Input: part model. Units: mm. Frame: model coordinates. Face numbers are marked on the shaded views. Round coordinates to 2 decimals unless told otherwise and drop trailing zeros. Order: outer loops, then holes, each group sorted by start corner. A loop starts at its lowest first (then second) coordinate and runs counter-clockwise, first axis right, second up. Notation, with made-up numbers: (17.25, -31.75) -> (44.25, -31.75) arc R16 cw to (44.25, -20.75) -> close; hole circle Ø11 at (-6.75, 20). An arc over 180 degrees is marked (long way). Answer as CSV lines item,"result". Start each with the question number.
1) Section query C-C, the plane x = 0. Output: boundary loops of the cut face in (y, z).
2) Section query A-A, the plane y = 2.75. Output: boundary loops of the cut face in (x, z).
3) Section query D-D, the plane z = 12. Output: boundary loops of the cut face in (x, y), and give its area (3 significant figures).
4) Line query: L1, parallel to Y at x = 0, z = -11.5; L2, parallel to Z at x = 0, y = -1; L3, parallel to X at y = 4.75, z = 15. Output: solid intervals per line, ascending.
5) Mould query, pull axis X, two halves, no side actions, for the marked faces 1, 2, 3 and 4. Classes: +X half, -X half, draft (parallel to the pull), parting line (faces both ways), or undercut.
6) Section query B-B, the plane z = -5.5. Output: boundary loops of the cut face in (x, y), and give its area (3 significant figures).
7) First-contact query: P1, Ø2, axis at x = 0.5, y = 1, coming from the -Z side; P2, Ø6.5, axis at x = 0, z = 15, coming from the -Y side. Flat tips, straight axial feed; report the tip coordinate or a pass-through.
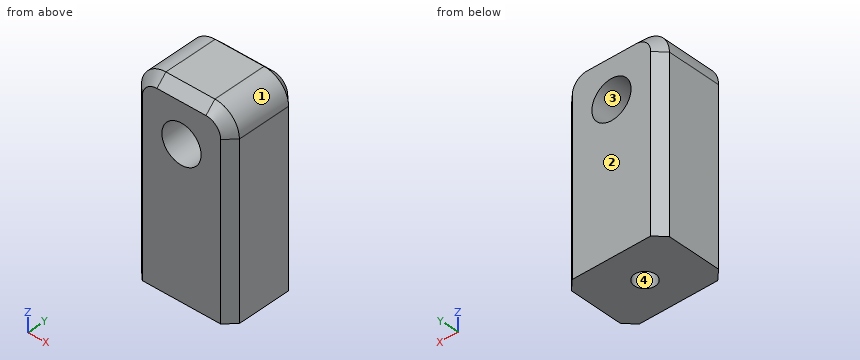
Autodesk Inventor part; units mm, degrees
ref_plane "YZ Plane" through (0, 0, 0) normal (1, 0, 0) x (0, 1, 0)
ref_plane "XZ Plane" through (0, 0, 0) normal (0, 1, 0) x (-1, 0, 0)
ref_plane "XY Plane" through (0, 0, 0) normal (0, 0, 1) x (1, 0, 0)
sketch "Sketch1" plane through (0, 0, 0) normal (0, 0, 1) x (1, 0, 0)
  line L0 (10, -7.5) -> (-10, -7.5)
  line L1 (-10, -7.5) -> (-10, 7.5)
  line L2 (-10, 7.5) -> (10, 7.5)
  line L3 (10, 7.5) -> (10, -7.5)
  line L4 (10, -7.5) -> (-10, 7.5) construction
  line L5 (-10, -7.5) -> (10, 7.5) construction
  line L6 (-10, 7.5) -> (10, 7.5)
  line L7 (10, 7.5) -> (10, 13.5)
  line L8 (10, 13.5) -> (-10, 13.5)
  line L9 (-10, 13.5) -> (-10, 7.5)
  line L10 (-10, -7.5) -> (10, -7.5)
  line L11 (10, -7.5) -> (10, -13.5)
  line L12 (10, -13.5) -> (-10, -13.5)
  line L13 (-10, -13.5) -> (-10, -7.5)
  point P0 (0, 0)
  dimension "d0" = 15
  dimension "d1" = 20
  dimension "d2" = 6
extrude "Extrusion1" add sketch "Sketch1" against normal blind 15
extrude "Extrusion2" add sketch "Sketch1" along normal blind 25 contours L11 L12 L13 L0 | L2 L9 L8 L7
sketch "Sketch2" plane through (-10, 13.5, -15) normal (0, 1, 0) x (1, 0, 0)
  line L0 (20, -15) -> (0, -15)
  line L1 (20, -40) -> (0, -40) construction
  line L2 (10, -40) -> (10, -30) construction
  circle A0 centre (10, -30) radius 4
  point P0 (10, -15)
  dimension "d7" = 8
  dimension "d8" = 10
extrude "Extrusion3" cut sketch "Sketch2" against normal through all
fillet "Fillet1" radius 5 4 edges at (-10, 10.5, 25) (10, 10.5, 25) (-10, -10.5, 25) (10, -10.5, 25)
sketch "Sketch3" plane through (0, 0, -15) normal (0, 0, -1) x (-1, 0, 0)
  circle A0 centre (0, 0) radius 2.15
  dimension "d12" = 4.3
extrude "Extrusion4" cut sketch "Sketch3" against normal through all
chamfer "Chamfer1" distance 2 angle 45 6 edges at (8.5355, 13.5, 23.5355) (0, 13.5, 25) (-8.5355, 13.5, 23.5355) (8.5355, -13.5, 23.5355) (0, -13.5, 25) (-8.5355, -13.5, 23.5355)
chamfer "Chamfer2" distance 4 angle 45 1 edges at (-10, 0, 0)
sketch "Sketch4" plane through (-5, 7.5, 25) normal (0, -1, 0) x (1, 0, 0)
  circle A0 centre (5, -10) radius 4
  arc A1 (15, -5) -> (10, 0) centre (10, -5) ccw
  line L0 (0, 0) -> (10, 0)
  arc A2 (0, 0) -> (-5, -5) centre (0, -5) ccw
  line L1 (-5, -29) -> (-5, -5)
  line L2 (-1, -25) -> (-5, -29)
  line L3 (15, -25) -> (-1, -25)
  line L4 (15, -25) -> (15, -5)
  point P0 (5, -25)
extrude "Extrusion5" add sketch "Sketch4" along normal up to next
sketch "Sketch5" plane through (0, 0, -15) normal (0, 0, -1) x (-1, 0, 0)
  line L0 (10, -11.5) -> (8, -13.5)
  line L1 (10, -11.5) -> (10, 11.5)
  line L2 (8, 13.5) -> (10, 11.5)
  line L3 (8, 13.5) -> (-8, 13.5)
  line L4 (-10, 11.5) -> (-8, 13.5)
  line L5 (-10, 11.5) -> (-10, -11.5)
  line L6 (-8, -13.5) -> (-10, -11.5)
  line L7 (-8, -13.5) -> (8, -13.5)
  circle A0 centre (0, 0) radius 2.15
  line L8 (-10, -11.5) -> (-10, 11.5)
  line L9 (-10, -7.5) -> (10, -7.5)
  line L10 (-10, 7.5) -> (10, 7.5)
  dimension "d23" = 6
  dimension "d24" = 6
extrude "Extrusion6" cut sketch "Sketch5" against normal through all contours L0 L7 L6 L5 L9 L1 | L10 L5 L4 L3 L2 L1
chamfer "Chamfer3" distance 2 angle 45 8 edges at (10, -7.5, 2.5) (0, -7.5, 25) (-10, -7.5, 2.5) (10, 7.5, 2.5) (8.5355, 7.5, 23.5355) (0, 7.5, 25) (-8.5355, 7.5, 23.5355) (-10, 7.5, 2.5)
properties part number "cylinder clevis 2"
Findings:
1,outline,"(-7.5, -15) -> (-2.15, -15) -> (-2.15, 0) -> (2.15, 0) -> (2.15, -15) -> (7.5, -15) -> (7.5, 11) -> (-7.5, 11) -> close; (-7.5, 19) -> (7.5, 19) -> (7.5, 23) -> (5.5, 25) -> (-5.5, 25) -> (-7.5, 23) -> close"
2,outline,"(-10, -15) -> (10, -15) -> (10, 20) arc R5 ccw to (5, 25) -> (-5, 25) arc R5 ccw to (-10, 20) -> close; hole circle Ø8 at (0, 15)"
3,outline,"(-10, -5.5) -> (-8, -7.5) -> (-2.65, -7.5) -> (-2.65, 7.5) -> (-8, 7.5) -> (-10, 5.5) -> close; (2.65, -7.5) -> (8, -7.5) -> (10, -5.5) -> (10, 5.5) -> (8, 7.5) -> (2.65, 7.5) -> close"
3,area,"213 mm^2"
4,L1,"y = -7.5 to -2.15, 2.15 to 7.5"
4,L2,"z = 0 to 11, 19 to 25"
4,L3,"x = -10 to -4, 4 to 10"
5,face 1,"+X half"
5,face 2,"draft"
5,face 3,"undercut"
5,face 4,"undercut"
6,outline,"(-10, -5.5) -> (-8, -7.5) -> (8, -7.5) -> (10, -5.5) -> (10, 5.5) -> (8, 7.5) -> (-8, 7.5) -> (-10, 5.5) -> close; hole circle Ø4.3 at (0, 0)"
6,area,"277 mm^2"
7,P1,"stops at z = 0"
7,P2,"passes through"
